Model file for the job. Use its own axes, mm. A direction names the side the tool comes from. Round coordinates to 2 decimals unless told otherwise and drop trailing zeros. Order: outer loops, then holes, each group sorted by start corner. A loop starts at its lowest first (then second) coordinate and runs counter-clockwise, first axis right, second up. Notation, with made-up numbers: (54.25, -25.5) - (80.25, -25.5) arc R23 ccw to (80.25, 7.5) - close; hole circle Ø2 at (84, -20). An arc over 180 degrees is marked (long way). Use one line per item in the form item = value.
from build123d import *

# Parameters (mm, degrees)
SKETCH_1_R          = 33.5
EXTRUDE_1_DEPTH     = 7
SKETCH_3_R          = 28.5
CUT_EXTRUDE_1_DEPTH = 5
SKETCH_4_R          = 2.5
CUT_EXTRUDE_2_DEPTH = 5
SKETCH_5_R          = 20
EXTRUDE_2_DEPTH     = 11
SKETCH_6_R          = 10
CUT_EXTRUDE_5_DEPTH = 10
M5X0_8_1_AT_2_COUNT = 2
M5X0_8_1_AT_2_PITCH = 31.5
M5X0_8_1_AT_3_COUNT = 2
M5X0_8_1_AT_3_PITCH = 22.273863607
M5X0_8_1_AT_4_COUNT = 2
M5X0_8_1_AT_4_PITCH = 22.273863607
SKETCH_7_R          = 2.5
CUT_EXTRUDE_6_DEPTH = 7


with BuildPart() as part:
    # ｽｹｯﾁ1 → 押し出し1 (new body)
    with BuildSketch(Plane(origin=(0, 0, 0), x_dir=(0, 0, -1), z_dir=(1, 0, 0))):
        Circle(SKETCH_1_R)
    extrude(amount=EXTRUDE_1_DEPTH)

    # ｽｹｯﾁ3 → ｶｯﾄ - 押し出し1 (cut)
    with BuildSketch(Plane(origin=(7, 0, 0), x_dir=(0, 0, -1), z_dir=(1, 0, 0))):
        Circle(SKETCH_3_R)
    extrude(amount=-CUT_EXTRUDE_1_DEPTH, mode=Mode.SUBTRACT)

    # ｽｹｯﾁ4 → ｶｯﾄ - 押し出し2 (cut)
    with BuildSketch(Plane(origin=(2, 0, 0), x_dir=(0, 0, -1), z_dir=(1, 0, 0))):
        Circle(SKETCH_4_R)
    extrude(amount=-CUT_EXTRUDE_2_DEPTH, mode=Mode.SUBTRACT)

    # ｽｹｯﾁ5 → 押し出し2 (add)
    with BuildSketch(Plane(origin=(2, 0, 0), x_dir=(0, 0, -1), z_dir=(1, 0, 0))):
        Circle(SKETCH_5_R)
    extrude(amount=EXTRUDE_2_DEPTH)

    # ｽｹｯﾁ6 → ｶｯﾄ - 押し出し5 (cut)
    with BuildSketch(Plane(origin=(13, 0, 0), x_dir=(0, 0, -1), z_dir=(1, 0, 0))):
        Circle(SKETCH_6_R)
    extrude(amount=-CUT_EXTRUDE_5_DEPTH, mode=Mode.SUBTRACT)

    # ｽｹｯﾁ10 → M5x0.8 ねじ穴1 (revolve, cut)
    with BuildSketch(Plane(origin=(13, 11.136931804, 11.136931804), x_dir=(0, 0, -1), z_dir=(0, 1, 0))):
        Polygon((0, 0), (0, 10.2618073), (2.1, 9), (2.1, 10), (2.5, 10), (2.5, 0), align=None)
    m5x0_8_1 = revolve(axis=Axis((19.35, 11.136931804, 11.136931804), (-1, 0, 0)), mode=Mode.SUBTRACT)

    # M5x0.8 ねじ穴1 at 2: M5x0.8 ねじ穴1 ×2
    with Locations(*[Vector(0, -0.7071067811865511, -0.707106781186544) * (i * M5X0_8_1_AT_2_PITCH) for i in range(1, M5X0_8_1_AT_2_COUNT)]):
        add(m5x0_8_1, mode=Mode.SUBTRACT)

    # M5x0.8 ねじ穴1 at 3: M5x0.8 ねじ穴1 ×2
    with Locations(*[(0, -i * M5X0_8_1_AT_3_PITCH, 0) for i in range(1, M5X0_8_1_AT_3_COUNT)]):
        add(m5x0_8_1, mode=Mode.SUBTRACT)

    # M5x0.8 ねじ穴1 at 4: M5x0.8 ねじ穴1 ×2
    with Locations(*[(0, 0, -i * M5X0_8_1_AT_4_PITCH) for i in range(1, M5X0_8_1_AT_4_COUNT)]):
        add(m5x0_8_1, mode=Mode.SUBTRACT)

    # ｽｹｯﾁ7 → ｶｯﾄ - 押し出し6 (cut)
    with BuildSketch(Plane(origin=(13, 0, 0), x_dir=(0, 0, -1), z_dir=(1, 0, 0))):
        with Locations((0, -15.740397433)):
            Circle(SKETCH_7_R)
    extrude(amount=-CUT_EXTRUDE_6_DEPTH, mode=Mode.SUBTRACT)


solid = part.part
(1) Pin check, flat tips, straight feed: pin 1 (4 mm diameter, centred on y = -16.5, z = -0.5, fed in from +X); pin 2 (1 mm diameter, centred on x = 6, y = -6.5, fed in from -Z); pin 3 (6 mm diameter, centred on x = 3, y = 13, fed in from +Z); pin 4 (6 mm diameter, centred on y = -2, z = 4.5, fed in from +X). Stop position of each tip, or through.
Report:
pin_1 = 13
pin_2 = -32.96
pin_3 = 31.97
pin_4 = 3
(2) Tool access for faces 1 (the face through (9.55, -18.18, 0.54)), 2 (the face through (1.01, -2.44, 0.54)): list every direction of +Z, -Z, +X, -X, +Y, -Y with a clear straight run to the whole face (end or side of a thin tool).
Report:
face_1 = +X
face_2 = -X
(3) Pull direction Z, two halves, no side cores. Call faces 3 (the face through (13, 9, 5)), 4 (the face through (8.07, -13.616, 11.462)), 5 (the face through (3, 9, -12)): released by +Z, released by -Z, zero draft, split by the parting line, or undercut.
Report:
face_3 = zero draft
face_4 = undercut
face_5 = undercut
(4) Slice it at C-C on x = 12. Give the cut face in (y, z).
Report:
outline = circle Ø40 at (0, 0); hole circle Ø5 at (-15.74, 0); hole circle Ø5 at (-11.14, -11.14); hole circle Ø5 at (-11.14, 11.14); hole circle Ø20 at (0, 0); hole circle Ø5 at (11.14, -11.14); hole circle Ø5 at (11.14, 11.14)
(5) Probe probe 1 along Y at (x, z) = (7.25, 0); probe 2 along Z at (x, y) = (5, 10.5); probe 3 along Z at (x, y) = (6.5, 6). List the from-to ranges inside material, lowest first. Write a range as [from, to].
Report:
probe_1 = [-20, -18.24], [-13.24, -10], [10, 20]
probe_2 = [-31.81, -26.5], [-17.02, -13.55], [-8.72, 8.72], [13.55, 17.02], [26.5, 31.81]
probe_3 = [-32.96, -27.86], [-19.08, -8], [8, 19.08], [27.86, 32.96]
(6) Slice it at B-B on y = 0. Give the cut face in (x, z), then the cut area to 3 significant figures.
Report:
outline = (0, -33.5) - (7, -33.5) - (7, -28.5) - (2, -28.5) - (2, -20) - (13, -20) - (13, -10) - (3, -10) - (3, 10) - (13, 10) - (13, 20) - (2, 20) - (2, 28.5) - (7, 28.5) - (7, 33.5) - (0, 33.5) - (0, 2.5) - (2, 2.5) - (2, -2.5) - (0, -2.5) - close
area = 414 mm2
(7) Slice it at D-D on y = -27.5. Give the cut face in (x, z).
Report:
outline = (0, -19.13) - (7, -19.13) - (7, -7.48) - (2, -7.48) - (2, 7.48) - (7, 7.48) - (7, 19.13) - (0, 19.13) - close
(8) Slice it at A-A on z = 0. Give the cut face in (x, y), then the cut area to 3 significant figures.
Report:
outline = (0, -33.5) - (7, -33.5) - (7, -28.5) - (2, -28.5) - (2, -20) - (13, -20) - (13, -18.24) - (6, -18.24) - (6, -13.24) - (13, -13.24) - (13, -10) - (3, -10) - (3, 10) - (13, 10) - (13, 20) - (2, 20) - (2, 28.5) - (7, 28.5) - (7, 33.5) - (0, 33.5) - (0, 2.5) - (2, 2.5) - (2, -2.5) - (0, -2.5) - close
area = 379 mm2
